Here's how the part is built. I have some questions about the finished solid (model axes, mm). A direction names the side the tool comes from. Round coordinates to 2 decimals unless told otherwise and drop trailing zeros. Loops run counter-clockwise (first coordinate to the right, second up) from the corner with the lowest first, then second, coordinate; pieces in that order, holes last. Notation, with made-up numbers: M 15,-21 L 22,-21 A14 cw 22,0 Z; hole C 63.25,8.25 d4. An arc over 180 degrees is marked long. Answer as a JSON object with one key per item and string values.
from build123d import *

# Parameters (mm, degrees)
BOSS_EXTRUDE1_DEPTH = 18
SKETCH4_W           = 12
SKETCH4_H           = 8
CUT_EXTRUDE1_DEPTH  = 2
FILLET1_R           = 10
FILLET2_R           = 0.5


with BuildPart() as part:
    # Sketch2 → Boss-Extrude1 (new body)
    with BuildSketch(Plane.XY):
        Polygon((21.637867966, 2.85), (18.937867966, 0.15), (-18.937867966, 0.15), (-21.637867966, 2.85), align=None)
    extrude(amount=-BOSS_EXTRUDE1_DEPTH)

    # Sketch4 → Cut-Extrude1 (cut)
    with BuildSketch(Plane.XZ.offset(-0.15)):
        with Locations((0, -7)):
            Rectangle(SKETCH4_W, SKETCH4_H)
    extrude(amount=-CUT_EXTRUDE1_DEPTH, mode=Mode.SUBTRACT)

    # Fillet1
    # the kernel refuses this fillet: 10 mm, written as the material it adds along each edge
    with BuildSketch(Plane(origin=(6, 2.15, -11), x_dir=(0, -1, 0), z_dir=(-1, 0, 0))) as fillet1_piece_1:
        with BuildLine():
            CenterArc((10, 6), FILLET1_R, 180, 36.869897646)
            Line((0, 6), (0, 0))
            Line((0, 0), (2, 0))
        make_face()
    extrude(amount=12)

    # Fillet2
    fillet2_edges = [part.edges().sort_by_distance(p)[0] for p in [
        (0, 2.15, -3),
    ]]
    fillet(fillet2_edges, radius=FILLET2_R)


solid = part.part
Item 1: We'd pull the mould along Z, two halves only. Please class faces 1 (the face through (0, 2, -18)), 2 (the face through (0, 2, 0)), 3 (the face through (0, 1, -3)): +Z half, -Z half, draft (parallel to the pull), parting line (faces both ways), or undercut.
Solution:
{"face 1": "-Z half", "face 2": "+Z half", "face 3": "undercut"}
Item 2: I want a section at D-D on z = -5.75. List the corners of the cut face in (x, y) for me, plus the area to 3 significant figures.
Solution:
{"outline": "M -21.64,2.85 L -18.94,0.15 L -6,0.15 L -6,2.12 L 6,2.12 L 6,0.15 L 18.94,0.15 L 21.64,2.85 Z", "area": "85.9 mm2"}
Item 3: For faces 4 (the face through (-20.27, 1.48, -8.87)), 5 (the face through (-6, 1, -6)), which set-ups out of +Z, -Z, +X, -X, +Y, -Y let a thin tool reach every point of the face, with its end or its side?
Solution:
{"face 4": "+Z, -Z, -X, -Y", "face 5": "-Y"}
Item 4: I want a section at A-A on y = 0.7. List the corners of the cut face in (x, z) for me, plus the area to 3 significant figures.
Solution:
{"outline": "M -19.49,-18 L 19.49,-18 L 19.49,0 L -19.49,0 Z; hole M -6,-10.19 L 6,-10.19 L 6,-3 L -6,-3 Z", "area": "615 mm2"}
Item 5: For P1, Ø0.8, axis at x = 2.5, z = -4.5, coming from the -Y side; P2, Ø1.6, axis at y = 1, z = -5.5, coming from the +X side, each with a flat end and sliding along its axis, tell me the tip position at first contact or that it passes through.
Solution:
{"P1": "stops at y = 2.15", "P2": "stops at x = 20.59"}
Item 6: I want a section at C-C on z = -8.5. List the corners of the cut face in (x, y) for me.
Solution:
{"outline": "M -21.64,2.85 L -18.94,0.15 L -6,0.15 L -6,1.52 L 6,1.52 L 6,0.15 L 18.94,0.15 L 21.64,2.85 Z"}
Item 7: I want a section at B-B on x = -1.5. List the corners of the cut face in (y, z) for me.
Solution:
{"outline": "M 0.15,-18 L 2.85,-18 L 2.85,0 L 0.15,0 L 0.15,-3 L 1.65,-3 A0.5 cw 2.15,-3.5 L 2.15,-5 A10 cw 0.15,-11 Z"}
Item 8: If I drill on L1, parallel to X at y = 1, z = -8.75; L2, parallel to X at y = 1.55, z = -8.25; L3, parallel to Y at x = -1.5, z = -6.25, over which ranges is the centre line in solid material (lowest first)? Write a range as from..to.
Solution:
{"L1": "x = -19.79..-6, 6..19.79", "L2": "x = -20.34..-6, 6..20.34", "L3": "y = 2.07..2.85"}
